Answer from the drawing. Dimensions are ordinates in mm from the lowest x, y and z of the part. A direction names the side the tool comes from. Coordinates: 2 decimals unless noted, no trailing zeros. Loops run counter-clockwise (first coordinate to the right, second up) from the corner with the lowest first, then second, coordinate; pieces in that order, holes last. Notation, with made-up numbers: (79.5, 33) -> (91.5, 33) arc R30 ccw to (91.5, 71) -> close; hole circle Ø9 at (55.25, 78). An arc over 180 degrees is marked (long way). Answer as CSV lines item,"result".
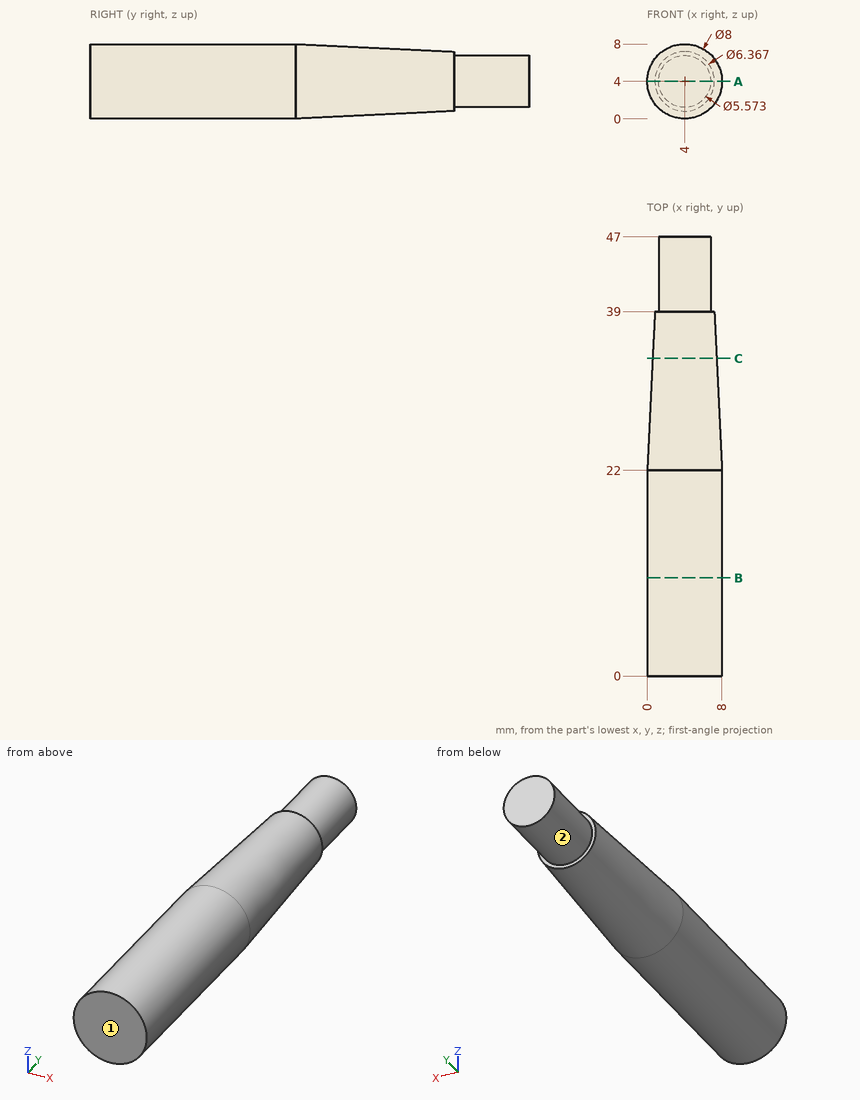
(1) Flat-ended cylindrical pins translate along their axes: pin 1 Ø2 at (x, y) = (6.5, 37.5) entering from -Z; pin 2 Ø1.5 at (x, y) = (7, 36) entering from -Z. Find the tip coordinate at first contact, or state that the pin passes through.
Computed values:
pin 1,"z = 1.11"
pin 2,"z = 1.55"
(2) A cutting plane is placed at A-A, the plane z = 4. Write down the section's boundary in (x, y), and give its area (3 significant figures).
Computed values:
outline,"(0, 0) -> (8, 0) -> (8, 22) -> (7.18, 39) -> (6.79, 39) -> (6.79, 47) -> (1.21, 47) -> (1.21, 39) -> (0.82, 39) -> (0, 22) -> close"
area,"343 mm2"
(3) Consider line 1 along Y through (x, z) = (6, 1.75); line 2 along X through (y, z) = (7.5, 3.75); line 3 along Z through (x, y) = (1.25, 25). Determine where each line is inside the solid, lowest interval first.
Computed values:
line 1,"0 to 39"
line 2,"0.01 to 7.99"
line 3,"1.3 to 6.7"
(4) A cutting plane is placed at B-B, the plane y = 10.5. Write down the section's boundary in (x, z), and give its area (3 significant figures).
Computed values:
outline,"circle Ø8 at (4, 4)"
area,"50.3 mm2"
(5) A cutting plane is placed at C-C, the plane y = 34. Write down the section's boundary in (x, z), and give its area (3 significant figures).
Computed values:
outline,"circle Ø6.85 at (4, 4)"
area,"36.8 mm2"
(6) Which of the six approach directions +Z, -Z, +X, -X, +Y, -Y give full straight-line access (tool end or side, diameter ignored) to the marked faces 1 and 2?
Computed values:
face 1,"+Z, -Z, +X, -X, -Y"
face 2,"+Y"
